```python
from build123d import *

# Parameters (mm, degrees)
F0_W     = 12.5
F0_H     = 8.5
F1_DEPTH = 4.5
F3_DEPTH = 3
F5_DEPTH = 12.5
F7_DEPTH = 12.5


with BuildPart() as f1:
    # F0 (on Top) → F1 (new body)
    with BuildSketch(Plane.XY):
        Rectangle(F0_W, F0_H)
    extrude(amount=F1_DEPTH)

    # F2 (on face) → F3 (join)
    with BuildSketch(Plane.XY.offset(4.5)):
        with BuildLine():
            add(Edge.make_bspline(
                [(-5, 3), (-3.3333333333, 3.2975326627), (0, 3.9024673373), (3.3333333333, 3.2975326627), (5, 3)],
                knots=[0, 0, 0, 0, 0.5, 1, 1, 1, 1], degree=3))
            Line((-5, 3), (-5, -3))
            add(Edge.make_bspline(
                [(-5, -3), (-3.3333333333, -3.2644556938), (0, -3.9355443062), (3.3333333333, -3.2644556938), (5, -3)],
                knots=[0, 0, 0, 0, 0.5, 1, 1, 1, 1], degree=3))
            Line((5, -3), (5, 3))
        make_face()
    extrude(amount=F3_DEPTH)

    # F4 (on Front) → F5 (cut, symmetric)
    with BuildSketch(Plane.XZ):
        with BuildLine():
            Line((5.0418378521, 7.7276835956), (-5.0418378521, 7.7276835956))
            Line((-5.0418378521, 7.7276835956), (-5.0418378521, 6.5))
            ThreePointArc((-5.0418378521, 6.5), (-4.1598718408, 7.2360679775), (-3.0418378521, 7.5))
            Line((-3.0418378521, 7.5), (3.0418378521, 7.5))
            ThreePointArc((3.0418378521, 7.5), (4.1598718408, 7.2360679775), (5.0418378521, 6.5))
            Line((5.0418378521, 6.5), (5.0418378521, 7.7276835956))
        make_face()
    extrude(amount=F5_DEPTH, both=True, mode=Mode.SUBTRACT)

    # F6 (on Right) → F7 (cut, symmetric)
    with BuildSketch(Plane.YZ):
        with BuildLine():
            Line((3.6354335025, 6), (3.6354335025, 7.9630231485))
            Line((3.6354335025, 7.9630231485), (-3.6354335025, 7.9630231485))
            Line((-3.6354335025, 7.9630231485), (-3.6354335025, 6))
            ThreePointArc((-3.6354335025, 6), (-3.1095768046, 7.0682118062), (-2, 7.5))
            Line((-2, 7.5), (2, 7.5))
            ThreePointArc((2, 7.5), (3.1095768046, 7.0682118062), (3.6354335025, 6))
        make_face()
    extrude(amount=F7_DEPTH, both=True, mode=Mode.SUBTRACT)


solid = f1.part
```
Check sheet for the modelled part. Datum: model origin and axes. Units: mm. A direction names the side the tool comes from. Round coordinates to 2 decimals unless told otherwise and drop trailing zeros. Order: outer loops, then holes, each group sorted by start corner. A loop starts at its lowest first (then second) coordinate and runs counter-clockwise, first axis right, second up. Notation, with made-up numbers: M 38,61 L 80,61 A29 cw 80,85 Z; hole C 17.5,24.25 d9. An arc over 180 degrees is marked long. Answer in a Markdown table with one row per item.
(1) Section check A-A on y = -1.75. Record the boundary of the cut face in (x, z).
Findings:
| item | result |
|---|---|
| outline | M -6.25,0 L 6.25,0 L 6.25,4.5 L 5,4.5 L 5,6.55 A2.5 ccw 3.04,7.5 L -3.04,7.5 A2.5 ccw -5,6.55 L -5,4.5 L -6.25,4.5 Z |
(2) Section check B-B on y = 2.25. Record the boundary of the cut face in (x, z).
Findings:
| item | result |
|---|---|
| outline | M -6.25,0 L 6.25,0 L 6.25,4.5 L 5,4.5 L 5,6.55 A2.5 ccw 3.35,7.48 L -3.35,7.48 A2.5 ccw -5,6.55 L -5,4.5 L -6.25,4.5 Z |
(3) Material ranges on line 1 along X through (y, z) = (-0.5, 5.25); line 2 along Z through (x, y) = (-5.25, -2); line 3 along Y through (x, z) = (-4.5, 6.25), recorded low to high. Write a range as from..to.
Findings:
| item | result |
|---|---|
| line 1 | x = -5..5 |
| line 2 | z = 0..4.5 |
| line 3 | y = -3.08..3.09 |
(4) Set-up check for faces 1 (the flat face through (-5, 0, 6)), 2 (the flat face through (5, 0, 6)), 3 (the flat face through (0, 0, 0)), 4 (the flat face through (0, -4, 4.5)): record each of +Z, -Z, +X, -X, +Y, -Y from which the full face is reachable in a straight line by a thin tool's end or side.
Findings:
| item | result |
|---|---|
| face 1 | +Z, -X, +Y, -Y |
| face 2 | +Z, +X, +Y, -Y |
| face 3 | -Z, +X, -X, +Y, -Y |
| face 4 | +Z |
(5) Gauge pin test, flat ends, axial feed: pin 1 (1.6 mm diameter, centred on y = -1.5, z = 6, fed in from -X); pin 2 (1.5 mm diameter, centred on x = 4, z = 5.5, fed in from +Y); pin 3 (1.6 mm diameter, centred on y = -1, z = 5.5, fed in from +X); pin 4 (4 mm diameter, centred on x = 1.5, y = -2.5, fed in from -Z). Record the tip position at first contact, or that the pin passes through.
Findings:
| item | result |
|---|---|
| pin 1 | stops at x = -5 |
| pin 2 | stops at y = 3.3 |
| pin 3 | stops at x = 5 |
| pin 4 | stops at z = 0 |
